```python
from build123d import *

# Parameters (mm, degrees)
F1_DEPTH      = 10
F2_SIZE       = 4
F4_W          = 20
F4_H          = 20.101140447
F5_DEPTH      = 3.3
F5_DEPTH_BACK = 3
F6_DEPTH      = 84
F7_SIZE       = 4
F8_R          = 1.75
F9_DEPTH      = 8.7
F10_R         = 1.65
F11_DEPTH     = 66.9
F12_R         = 2.4
F13_DEPTH     = 25


with BuildPart() as f1:
    # F0 (on Front) → F1 (new body, symmetric)
    with BuildSketch(Plane.XZ):
        Polygon((-22.3, 4.5), (-27, 4.5), (-27, -3.4), (-25.5, -3.4), (-25.5, -15.4), (-9.5, -15.4), (-9.5, 0), (16.8, 0), (16.8, -5), (27, -5), (27, 0), (27, 4.5), (-2.3, 4.5), (-2.3, 12.5), (-22.3, 12.5), align=None)
    extrude(amount=F1_DEPTH, both=True)

    # F2
    f2_edges = [f1.edges().sort_by_distance(p)[0] for p in [
        (-17.5, -10, -15.4),
        (-17.5, 10, -15.4),
    ]]
    chamfer(f2_edges, length=F2_SIZE)

    # F4 (on face) → F5 (join, two sides)
    with BuildSketch(Plane.YZ.offset(27)) as f5_sk:
        with Locations((0, -5.5505702235)):
            Rectangle(F4_W, F4_H)
    extrude(amount=F5_DEPTH)
    extrude(f5_sk.sketch, amount=-F5_DEPTH_BACK)

    # F3 (on face) → F6 (cut)
    with BuildSketch(Plane(origin=(-25.5, 0, 0), x_dir=(0, -1, 0), z_dir=(-1, 0, 0))):
        with BuildLine():
            ThreePointArc((4.1, -9.4), (2.8991378029, -6.5008621971), (0, -5.3))
            Line((0, -5.3), (0, -13.5))
            ThreePointArc((0, -13.5), (2.8991378029, -12.2991378029), (4.1, -9.4))
        make_face()
        with BuildLine():
            Line((0, -13.5), (0, -5.3))
            ThreePointArc((0, -5.3), (-4.1, -9.4), (0, -13.5))
        make_face()
    extrude(amount=-F6_DEPTH, mode=Mode.SUBTRACT)

    # F7
    f7_edges = [f1.edges().sort_by_distance(p)[0] for p in [
        (27.15, 10, -15.60114),
        (27.15, -10, -15.60114),
    ]]
    chamfer(f7_edges, length=F7_SIZE)

    # F8 (on face) → F9 (cut)
    with BuildSketch(Plane.XZ.offset(10)):
        with Locations((27.2387061268, -9.3012042344)):
            Circle(F8_R)
    extrude(amount=-F9_DEPTH, mode=Mode.SUBTRACT)

    # F10 (on face) → F11 (cut)
    with BuildSketch(Plane.YZ.offset(30.3)):
        with Locations((5.1269349642, 8.461603526)):
            Circle(F10_R)
        with Locations((-5.1269349642, 8.461603526)):
            Circle(F10_R)
    extrude(amount=-F11_DEPTH, mode=Mode.SUBTRACT)

    # F12 (on face) → F13 (cut)
    with BuildSketch(Plane(origin=(0, 10, 0), x_dir=(-1, 0, 0), z_dir=(0, 1, 0))):
        with Locations((21.0122950375, -8.7536005303)):
            Circle(F12_R)
        with Locations((13.9877049625, -8.7536005303)):
            Circle(F12_R)
    extrude(amount=-F13_DEPTH, mode=Mode.SUBTRACT)


solid = f1.part
```
Verification items for the finished model (mm, model axes). A direction names the side the tool comes from. Coordinates: 2 decimals unless noted, no trailing zeros. Loops run counter-clockwise (first coordinate to the right, second up) from the corner with the lowest first, then second, coordinate; pieces in that order, holes last. Notation, with made-up numbers: (53.25, 71.5) -> (112.25, 71.5) arc R25 cw to (112.25, 85.5) -> close; hole circle Ø10 at (62.25, 64.5). An arc over 180 degrees is marked (long way). Answer in a Markdown table with one row per item. Add a question column.
1. Section check C-C, the plane y = 1.75. Enter the section's corners in (x, z).
2. Section check D-D, the plane y = 8. Enter the section's corners in (x, z).
3. Material ranges on probe 1 along X at (y, z) = (6.75, -3); probe 2 along Z at (x, y) = (-13, 5.5); probe 3 along X at (y, z) = (4, -6), recorded low to high. Write a range as [from, to].
4. Section check B-B, the plane y = -8. Enter the section's corners in (x, z), then the cut area to 3 significant figures.
5. Depth check by flat-ended pin: P1, Ø2.5, axis at y = -4.5, z = 10.5, coming from the -X side; P2, Ø2, axis at x = 20, y = -3, coming from the -Z side; P3, Ø10, axis at x = 10, y = -2, coming from the -Z side. Enter the tip coordinate at first touch or a pass-through.
6. Access from +Z, -Z, +X, -X, +Y, -Y to the whole of each face (thin tool, end or side, straight path). Record for faces 4 (the face through (16.8, 0, -2)), 5 (the face through (-25.5, 2, -5)), 6 (the face through (-25, 0, 4.5)).
7. Draft check along X on faces 1 (the face through (-27, 0, 1)), 2 (the face through (-18, 0, -15.4)), 3 (the face through (-15.28, 7.23, -6.73)). Enter one of: +X half, -X half, draft (parallel to the pull), parting line (faces both ways), or undercut.
8. Section check A-A, the plane z = -1. Enter the section's corners in (x, y), then the cut area to 3 significant figures.
Derived:
| question | item | result |
|---|---|---|
| 1 | outline | (-27, -3.4) -> (-25.5, -3.4) -> (-25.5, -5.69) -> (-9.5, -5.69) -> (-9.5, 0) -> (16.8, 0) -> (16.8, -5) -> (24, -5) -> (24, -5.69) -> (30.3, -5.69) -> (30.3, 4.5) -> (-2.3, 4.5) -> (-2.3, 12.5) -> (-22.3, 12.5) -> (-22.3, 4.5) -> (-27, 4.5) -> close; (-25.5, -15.4) -> (-9.5, -15.4) -> (-9.5, -13.11) -> (-25.5, -13.11) -> close; (24, -15.6) -> (30.3, -15.6) -> (30.3, -13.11) -> (24, -13.11) -> close |
| 2 | outline | (-27, -3.4) -> (-25.5, -3.4) -> (-25.5, -13.4) -> (-9.5, -13.4) -> (-9.5, 0) -> (16.8, 0) -> (16.8, -5) -> (24, -5) -> (24, -13.6) -> (30.3, -13.6) -> (30.3, 4.5) -> (-2.3, 4.5) -> (-2.3, 12.5) -> (-22.3, 12.5) -> (-22.3, 4.5) -> (-27, 4.5) -> close; hole circle Ø4.8 at (-21.01, -8.75); hole circle Ø4.8 at (-13.99, -8.75) |
| 3 | probe 1 | x = [-27, -9.5], [16.8, 30.3] |
| 3 | probe 2 | z = [-15.4, -10.94], [-6.57, 6.85], [10.07, 12.5] |
| 3 | probe 3 | x = [-25.5, -9.5], [24, 30.3] |
| 4 | outline | (-27, -3.4) -> (-25.5, -3.4) -> (-25.5, -13.4) -> (-9.5, -13.4) -> (-9.5, 0) -> (16.8, 0) -> (16.8, -5) -> (24, -5) -> (24, -13.6) -> (30.3, -13.6) -> (30.3, 4.5) -> (-2.3, 4.5) -> (-2.3, 12.5) -> (-22.3, 12.5) -> (-22.3, 4.5) -> (-27, 4.5) -> close; hole circle Ø4.8 at (-21.01, -8.75); hole circle Ø4.8 at (-13.99, -8.75); hole circle Ø3.5 at (27.24, -9.3) |
| 4 | area | 713 mm² |
| 5 | P1 | stops at x = -22.3 |
| 5 | P2 | stops at z = -5 |
| 5 | P3 | stops at z = 0 |
| 6 | face 4 | -Z, +Y, -Y |
| 6 | face 5 | -Z, -X, +Y, -Y |
| 6 | face 6 | +Z, -X, +Y, -Y |
| 7 | face 1 | -X half |
| 7 | face 2 | draft |
| 7 | face 3 | undercut |
| 8 | outline | (-27, -10) -> (-9.5, -10) -> (-9.5, 10) -> (-27, 10) -> close; (16.8, -10) -> (30.3, -10) -> (30.3, 10) -> (16.8, 10) -> close |
| 8 | area | 620 mm² |
